The listing builds one solid part. Answer for the finished solid, in the listing's coordinates (mm). Face numbers are marked on the shaded views. A direction names the side the tool comes from. Give positions to 0.01 mm unless a question says otherwise; leave off trailing zeros. Write each loop counter-clockwise with the first axis right and the second up, starting at its lowest first coordinate (ties: lowest second). Pieces come first, ordered by that corner, then holes. Notation, with made-up numbers: M 17.25,-18.75 L 57.25,-18.75 A33 ccw 57.25,13.25 Z; hole C -18.75,32.25 d3. An arc over 180 degrees is marked long. Answer as a JSON object with one key per item and string values.
```python
from build123d import *

# Parameters (mm, degrees)
F0_R     = 7.5
F3_DEPTH = 33
F5_START = 3
F4_R     = 42
F5_DEPTH = 30


with BuildPart() as f2:
    # F1 (on Front) → F2 (revolve)
    with BuildSketch(Plane.XZ):
        with BuildLine():
            Line((-32.6045845728, 47.1321178182), (-42.5, 33))
            Line((-42.5, 33), (-26, 33))
            Line((-26, 33), (-26, 63))
            Line((-26, 63), (-29, 63))
            Line((-29, 63), (-37, 93))
            Line((-37, 93), (-45, 93))
            Line((-45, 93), (-45, 85))
            Line((-45, 85), (-50, 85))
            Line((-50, 85), (-50, 55))
            Line((-50, 55), (-36.7003447942, 55))
            ThreePointArc((-36.7003447942, 55), (-32.2652906284, 52.3087430662), (-32.6045845728, 47.1321178182))
        make_face()
    revolve(axis=Axis((0, 0, 36.171267882), (0, 0, 1)))

    # F0 (on Top) → F3 (join)
    with BuildSketch(Plane.XY):
        with BuildLine():
            ThreePointArc((30.7416238862, 32.8626316785), (38.4714348159, 23.3441363774), (43.3448275862, 12.0923910589))
            ThreePointArc((43.3448275862, 12.0923910589), (53.6337221418, 18.491501228), (65.6982762183, 17.3705654274))
            Line((65.6982762183, 17.3705654274), (30.7416238862, 32.8626316785))
        make_face()
        with BuildLine():
            ThreePointArc((-43.3448275862, 12.0923910589), (-38.4714348159, 23.3441363774), (-30.7416238862, 32.8626316785))
            Line((-30.7416238862, 32.8626316785), (-65.6982778503, 17.3705647041))
            ThreePointArc((-65.6982778503, 17.3705647041), (-53.6337230105, 18.4915014331), (-43.3448275862, 12.0923910589))
        make_face()
        with BuildLine():
            Line((-65.6982756625, -17.3705656737), (-30.7416238862, -32.8626316785))
            ThreePointArc((-30.7416238862, -32.8626316785), (-38.4714348159, -23.3441363774), (-43.3448275862, -12.0923910589))
            ThreePointArc((-43.3448275862, -12.0923910589), (-53.633721846, -18.4915011581), (-65.6982756625, -17.3705656737))
        make_face()
        with BuildLine():
            ThreePointArc((65.6982756625, -17.3705656737), (53.633721846, -18.4915011582), (43.3448275862, -12.0923910589))
            ThreePointArc((43.3448275862, -12.0923910589), (38.4714348159, -23.3441363774), (30.7416238862, -32.8626316785))
            Line((30.7416238862, -32.8626316785), (65.6982756625, -17.3705656737))
        make_face()
        with BuildLine():
            ThreePointArc((41.4590517241, 9.3486378759), (42.3417264073, 10.7618989076), (43.3448275862, 12.0923910589))
            ThreePointArc((43.3448275862, 12.0923910589), (38.4714348159, 23.3441363774), (30.7416238862, 32.8626316785))
            Line((30.7416238862, 32.8626316785), (17.219827087, 38.8552127146))
            ThreePointArc((17.219827087, 38.8552127146), (32.8399481472, 26.9775426177), (41.4590517241, 9.3486378759))
        make_face()
        with BuildLine():
            Line((-17.2198272904, 38.8552126244), (-30.7416238862, 32.8626316785))
            ThreePointArc((-30.7416238862, 32.8626316785), (-38.4714348159, 23.3441363774), (-43.3448275862, 12.0923910589))
            ThreePointArc((-43.3448275862, 12.0923910589), (-42.3417264073, 10.7618989076), (-41.4590517241, 9.3486378759))
            ThreePointArc((-41.4590517241, 9.3486378759), (-32.8399482178, 26.9775425317), (-17.2198272904, 38.8552126244))
        make_face()
        with BuildLine():
            ThreePointArc((-43.3448275862, -12.0923910589), (-45, 0), (-43.3448275862, 12.0923910589))
            ThreePointArc((-43.3448275862, 12.0923910589), (-53.6337230105, 18.4915014331), (-65.6982778503, 17.3705647041))
            ThreePointArc((-65.6982778503, 17.3705647041), (-77, -1.1965e-06), (-65.6982756625, -17.3705656737))
            ThreePointArc((-65.6982756625, -17.3705656737), (-53.633721846, -18.4915011581), (-43.3448275862, -12.0923910589))
        make_face()
        with Locations((-58, 0)):
            Circle(F0_R, mode=Mode.SUBTRACT)
        with BuildLine():
            ThreePointArc((-43.3448275862, -12.0923910589), (-38.4714348159, -23.3441363774), (-30.7416238862, -32.8626316785))
            Line((-30.7416238862, -32.8626316785), (-17.2198274837, -38.8552125388))
            ThreePointArc((-17.2198274837, -38.8552125388), (-32.8399482849, -26.9775424501), (-41.4590517241, -9.3486378759))
            ThreePointArc((-41.4590517241, -9.3486378759), (-42.3417264073, -10.7618989076), (-43.3448275862, -12.0923910589))
        make_face()
        with BuildLine():
            ThreePointArc((30.7416238862, -32.8626316785), (38.4714348159, -23.3441363774), (43.3448275862, -12.0923910589))
            ThreePointArc((43.3448275862, -12.0923910589), (42.3417264073, -10.7618989076), (41.4590517241, -9.3486378759))
            ThreePointArc((41.4590517241, -9.3486378759), (32.8399481447, -26.9775426208), (17.2198270797, -38.8552127178))
            Line((17.2198270797, -38.8552127178), (30.7416238862, -32.8626316785))
        make_face()
        with BuildLine():
            ThreePointArc((43.3448275862, 12.0923910589), (44.5842867016, 6.1025715326), (45, 0))
            ThreePointArc((45, 0), (44.5842867016, -6.1025715326), (43.3448275862, -12.0923910589))
            ThreePointArc((43.3448275862, -12.0923910589), (53.633721846, -18.4915011582), (65.6982756625, -17.3705656737))
            ThreePointArc((65.6982756625, -17.3705656737), (73.9258789018, -10.3617750027), (77, 0))
            ThreePointArc((77, 0), (73.9258790675, 10.3617747479), (65.6982762183, 17.3705654274))
            ThreePointArc((65.6982762183, 17.3705654274), (53.6337221418, 18.491501228), (43.3448275862, 12.0923910589))
        make_face()
        with Locations((58, 0)):
            Circle(F0_R, mode=Mode.SUBTRACT)
        with BuildLine():
            ThreePointArc((43.3448275862, -12.0923910589), (44.5842867016, -6.1025715326), (45, 0))
            ThreePointArc((45, 0), (44.5842867016, 6.1025715326), (43.3448275862, 12.0923910589))
            ThreePointArc((43.3448275862, 12.0923910589), (42.3417264073, 10.7618989076), (41.4590517241, 9.3486378759))
            ThreePointArc((41.4590517241, 9.3486378759), (42.2389612696, 4.7032064448), (42.5, 0))
            ThreePointArc((42.5, 0), (42.2389612696, -4.7032064448), (41.4590517241, -9.3486378759))
            ThreePointArc((41.4590517241, -9.3486378759), (42.3417264073, -10.7618989076), (43.3448275862, -12.0923910589))
        make_face()
        with BuildLine():
            ThreePointArc((-41.4590517241, 9.3486378759), (-42.3417264073, 10.7618989076), (-43.3448275862, 12.0923910589))
            ThreePointArc((-43.3448275862, 12.0923910589), (-45, 0), (-43.3448275862, -12.0923910589))
            ThreePointArc((-43.3448275862, -12.0923910589), (-42.3417264073, -10.7618989076), (-41.4590517241, -9.3486378759))
            ThreePointArc((-41.4590517241, -9.3486378759), (-42.5, 0), (-41.4590517241, 9.3486378759))
        make_face()
        with BuildLine():
            ThreePointArc((17.2198270797, -38.8552127178), (32.8399481447, -26.9775426208), (41.4590517241, -9.3486378759))
            ThreePointArc((41.4590517241, -9.3486378759), (41.2735245316, -9.0124923526), (41.0948275862, -8.672666583))
            ThreePointArc((41.0948275862, -8.672666583), (0, -42), (-41.0948275862, -8.672666583))
            ThreePointArc((-41.0948275862, -8.672666583), (-41.2735245316, -9.0124923526), (-41.4590517241, -9.3486378759))
            ThreePointArc((-41.4590517241, -9.3486378759), (-32.8399482849, -26.9775424501), (-17.2198274837, -38.8552125388))
            ThreePointArc((-17.2198274837, -38.8552125388), (-2.209e-07, -42.5), (17.2198270797, -38.8552127178))
        make_face()
        with BuildLine():
            ThreePointArc((41.0948275862, 8.672666583), (41.2735245316, 9.0124923526), (41.4590517241, 9.3486378759))
            ThreePointArc((41.4590517241, 9.3486378759), (32.8399481472, 26.9775426177), (17.219827087, 38.8552127146))
            ThreePointArc((17.219827087, 38.8552127146), (-1.113e-07, 42.5), (-17.2198272904, 38.8552126244))
            ThreePointArc((-17.2198272904, 38.8552126244), (-32.8399482178, 26.9775425317), (-41.4590517241, 9.3486378759))
            ThreePointArc((-41.4590517241, 9.3486378759), (-41.2735245316, 9.0124923526), (-41.0948275862, 8.672666583))
            ThreePointArc((-41.0948275862, 8.672666583), (0, 42), (41.0948275862, 8.672666583))
        make_face()
        with BuildLine():
            ThreePointArc((42.5, 0), (42.2389612696, 4.7032064448), (41.4590517241, 9.3486378759))
            ThreePointArc((41.4590517241, 9.3486378759), (41.2735245316, 9.0124923526), (41.0948275862, 8.672666583))
            ThreePointArc((41.0948275862, 8.672666583), (41.7730939638, 4.3598876923), (42, 0))
            ThreePointArc((42, 0), (41.7730939638, -4.3598876923), (41.0948275862, -8.672666583))
            ThreePointArc((41.0948275862, -8.672666583), (41.2735245316, -9.0124923526), (41.4590517241, -9.3486378759))
            ThreePointArc((41.4590517241, -9.3486378759), (42.2389612696, -4.7032064448), (42.5, 0))
        make_face()
        with BuildLine():
            ThreePointArc((-41.0948275862, -8.672666583), (-42, 0), (-41.0948275862, 8.672666583))
            ThreePointArc((-41.0948275862, 8.672666583), (-41.2735245316, 9.0124923526), (-41.4590517241, 9.3486378759))
            ThreePointArc((-41.4590517241, 9.3486378759), (-42.5, 0), (-41.4590517241, -9.3486378759))
            ThreePointArc((-41.4590517241, -9.3486378759), (-41.2735245316, -9.0124923526), (-41.0948275862, -8.672666583))
        make_face()
    extrude(amount=F3_DEPTH)

    # F4 (on Top) → F5 (join)
    with BuildSketch(Plane.XY.offset(F5_START)):
        Circle(F4_R)
    extrude(amount=F5_DEPTH)


solid = f2.part
```
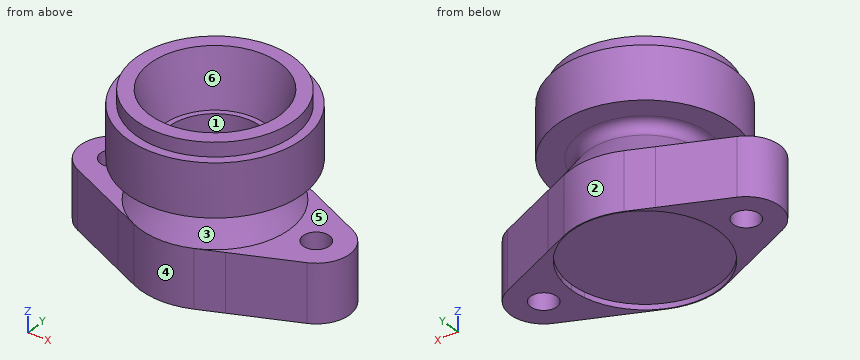
1. A cutting plane is placed at B-B, the plane z = 8. Give the vertices of the cut face in (x, y), plus the area to 3 significant figures.
Verdict:
{"outline": "M -65.7,-17.37 L -17.22,-38.86 A42.5 ccw 17.22,-38.86 L 65.7,-17.37 A19 ccw 65.7,17.37 L 17.22,38.86 A42.5 ccw -17.22,38.86 L -65.7,17.37 A19 ccw Z; hole C -58,0 d15; hole C 58,0 d15", "area": "8,510 mm2"}
2. The mould has two halves that part along Z. Classify the marked faces 4, 5 and 6: released by +Z, released by -Z, zero draft, split by the parting line, or undercut.
Verdict:
{"face 4": "zero draft", "face 5": "undercut", "face 6": "released by +Z"}
3. A cutting plane is placed at D-D, the plane x = 58.5. Give the vertices of the cut face in (y, z), plus the area to 3 significant figures.
Verdict:
{"outline": "M -20.56,0 L -7.48,0 L -7.48,33 L -20.56,33 Z; M 7.48,0 L 20.56,0 L 20.56,33 L 7.48,33 Z", "area": "863 mm2"}
4. A cutting plane is placed at C-C, the plane z = 45. Give the vertices of the cut face in (x, y), plus the area to 3 significant figures.
Verdict:
{"outline": "C 0,0 d68.2; hole C 0,0 d52", "area": "1,530 mm2"}
5. Consider line 1 along Z through (x, y) = (23, -1.5); line 2 along X through (y, z) = (5, 71.5); line 3 along Y through (x, z) = (58, 13). Determine where each line is inside the solid, lowest interval first.
Verdict:
{"line 1": "z = 3 to 33", "line 2": "x = -49.75 to -30.86, 30.86 to 49.75", "line 3": "y = -20.78 to -7.5, 7.5 to 20.78"}
6. For the marked faces 1, 2 and 3, determine the directions among +Z, -Z, +X, -X, +Y, -Y from which every point of the face is accessible in a straight line to the end or side of a thin tool.
Verdict:
{"face 1": "+Z", "face 2": "-Z, +Y", "face 3": "none"}
7. Flat-ended cylindrical pins translate along their axes: pin 1 (1 mm diameter, centred on x = 55, z = 11.5, fed in from -Y); pin 2 (8 mm diameter, centred on x = 6, y = -10.5, fed in from +Z); pin 3 (1.5 mm diameter, centred on x = -18.5, z = 43.5, fed in from +Y); pin 4 (12 mm diameter, centred on x = 58, y = 0, fed in from -Z). Find the tip coordinate at first contact, or state that the pin passes through.
Verdict:
{"pin 1": "stops at y = -22.33", "pin 2": "stops at z = 33", "pin 3": "stops at y = 30.65", "pin 4": "passes through"}
8. A cutting plane is placed at A-A, the plane x = -53. Give the vertices of the cut face in (y, z), plus the area to 3 significant figures.
Verdict:
{"outline": "M -23,0 L -5.59,0 L -5.59,33 L -23,33 Z; M 5.59,0 L 23,0 L 23,33 L 5.59,33 Z", "area": "1,150 mm2"}
